Build history of the part. All positions in model axes, mm. A direction names the side the tool comes from. Coordinates: 2 decimals unless noted, no trailing zeros. Order: outer loops, then holes, each group sorted by start corner. A loop starts at its lowest first (then second) coordinate and runs counter-clockwise, first axis right, second up. Notation, with made-up numbers: (70, -7) - (101, -7) arc R6 ccw to (101, -2) - close; hole circle Ø3 at (41.5, -8). An arc over 180 degrees is marked (long way). Return JSON: item names as keys, results as strings.
from build123d import *

# Parameters (mm, degrees)
ESQUISSE1_R        = 2.15
BOSS_EXTRU_1_DEPTH = 1.85
ESQUISSE2_R        = 1.25
BOSS_EXTRU_2_DEPTH = 4
CHANFREIN1_SIZE    = 1.85
CHANFREIN1_SIZE_2  = 0.15
CONG_1_R           = 0.1


with BuildPart() as part:
    # Esquisse1 → Boss.-Extru.1 (new body)
    with BuildSketch(Plane(origin=(0, 0, 0), x_dir=(1, 0, 0), z_dir=(0, 1, 0))):
        with Locations(Location((0, 0, 0), (0, 0, 270))):
            Circle(ESQUISSE1_R)
    extrude(amount=BOSS_EXTRU_1_DEPTH)

    # Esquisse2 → Boss.-Extru.2 (add)
    with BuildSketch(Plane(origin=(0, 1.85, 0), x_dir=(1, 0, 0), z_dir=(0, 1, 0))):
        with Locations(Location((0, 0, 0), (0, 0, 270))):
            Circle(ESQUISSE2_R)
    extrude(amount=BOSS_EXTRU_2_DEPTH)

    # Chanfrein1
    # the kernel refuses this chamfer: 1.85, 0.15 mm, written as the material it takes off along each edge
    with BuildSketch(Plane(origin=(0, 0, 0), x_dir=(0, 0, 1), z_dir=(-1, 0, 0))) as chanfrein1_piece_1:
        Polygon((2.15, CHANFREIN1_SIZE), (2.15 - CHANFREIN1_SIZE_2, 0), (2.15, 0), align=None)
    revolve(axis=Axis((0, 0, 0), (0, 1, 0)), mode=Mode.SUBTRACT)

    # Congé1
    cong_1_edges = [part.edges().sort_by_distance(p)[0] for p in [
        (0, 0, -2),
    ]]
    fillet(cong_1_edges, radius=CONG_1_R)


solid = part.part
1. Cut at B-B on z = 0. Give the cut face in (x, y), plus the area to 3 significant figures.
Check values:
{"outline": "(-2.15, 1.85) - (-2.01, 0.09) arc R0.1 ccw to (-1.91, 0) - (1.91, 0) arc R0.1 ccw to (2.01, 0.09) - (2.15, 1.85) - (1.25, 1.85) - (1.25, 5.85) - (-1.25, 5.85) - (-1.25, 1.85) - close", "area": "17.7 mm²"}
2. Cut at A-A on x = 0. Give the cut face in (y, z), plus the area to 3 significant figures.
Check values:
{"outline": "(0, -1.91) arc R0.1 ccw to (0.09, -2.01) - (1.85, -2.15) - (1.85, -1.25) - (5.85, -1.25) - (5.85, 1.25) - (1.85, 1.25) - (1.85, 2.15) - (0.09, 2.01) arc R0.1 ccw to (0, 1.91) - close", "area": "17.7 mm²"}
3. Drop flat-ended pins along their axis: pin 1 (1.5 mm diameter, centred on x = 1, y = 1.5, fed in from +Z); pin 2 (1 mm diameter, centred on x = 1.5, y = 0.5, fed in from -Z). Give the stop position or say it passes through.
Check values:
{"pin 1": "z = 2.12", "pin 2": "z = -1.78"}
4. Probe L1, parallel to Y at x = -1, z = -1.3; L2, parallel to X at y = 5.25, z = -0.5; L3, parallel to Z at x = -0.3, y = 3.35. List the from-to ranges inside material, lowest first.
Check values:
{"L1": "0 to 1.85", "L2": "-1.15 to 1.15", "L3": "-1.21 to 1.21"}
5. Cut at D-D on y = 0.55. Give the cut face in (x, z).
Check values:
{"outline": "circle Ø4.09 at (0, 0)"}
6. Cut at C-C on y = 2.6. Give the cut face in (x, z).
Check values:
{"outline": "circle Ø2.5 at (0, 0)"}
7. Tool access for faces 1 (the conical face through (-2.01, 0.76, -0.45)), 2 (the flat face through (-1, 1.85, 1)): list every direction of +Z, -Z, +X, -X, +Y, -Y with a clear straight run to the whole face (end or side of a thin tool).
Check values:
{"face 1": "-Y", "face 2": "+Y"}
